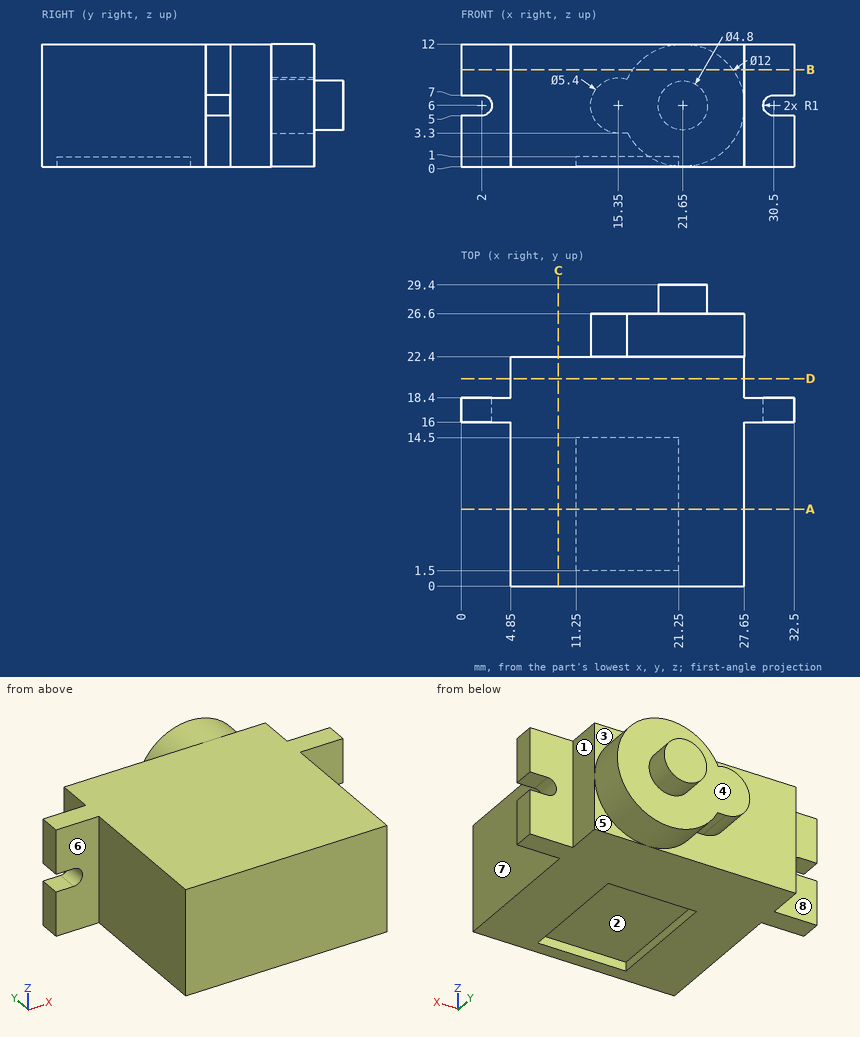
Study the drawing (mm; zero at the part's minimum x, y, z) and answer. A direction names the side the tool comes from. Coordinates: 2 decimals unless noted, no trailing zeros. Loops run counter-clockwise (first coordinate to the right, second up) from the corner with the lowest first, then second, coordinate; pieces in that order, holes last. Notation, with made-up numbers: M 69.5,74.5 L 124.5,74.5 A23 cw 124.5,106.5 Z; hole C 41.25,-24 d4. An arc over 180 degrees is marked long. Answer as a JSON object with one key per item and string values. Group by question number.
Item 1: Consider L1, parallel to Y at x = 16.5, z = 0.5; L2, parallel to Y at x = 14, z = 9.5; L3, parallel to Y at x = 17.5, z = 4. Determine where each line is inside the solid, lowest interval first.
Item 2: Each of these flat-tipped pins is pushed along its axis until it touches: P1, Ø1.8, axis at x = 25.5, z = 8.5, coming from the +Y side; P2, Ø5, axis at x = 22, z = 10, coming from the -Y side; P3, Ø5.5, axis at x = 3.5, z = 4.5, coming from the +Y side; P4, Ø1.5, axis at y = 21, z = 9, coming from the -X side. Where does it stop, or does it pass through?
Item 3: Section B-B (z = 9.5) is taken. Write down the section's boundary in (x, y), and give its area (3 significant figures).
Item 4: Section A-A (y = 7.5) is taken. Write down the section's boundary in (x, z), and give its area (3 significant figures).
Item 5: Section D-D (y = 20.25) is taken. Write down the section's boundary in (x, z).
Item 6: Determine the mould class of the marked faces 1, 2 and 3 for opening direction Y: +Y half, -Y half, draft (parallel to the pull), parting line (faces both ways), or undercut.
Item 7: Section C-C (x = 9.5) is taken. Write down the section's boundary in (y, z).
Item 8: Which of the six approach directions +Z, -Z, +X, -X, +Y, -Y give full straight-line access (tool end or side, diameter ignored) to the marked faces 4, 5, 6, 7 and 8?
Solved:
{
 "1": {"L1": "y = 0 to 1.5, 14.5 to 22.4", "L2": "y = 0 to 22.4", "L3": "y = 0 to 26.6"},
 "2": {"P1": "stops at y = 26.6", "P2": "stops at y = 0", "P3": "stops at y = 22.4", "P4": "stops at x = 4.85"},
 "3": {"outline": "M 0,16 L 4.85,16 L 4.85,0 L 27.65,0 L 27.65,16 L 32.5,16 L 32.5,18.4 L 27.65,18.4 L 27.65,22.4 L 26.52,22.4 L 26.52,26.6 L 16.78,26.6 L 16.78,22.4 L 4.85,22.4 L 4.85,18.4 L 0,18.4 Z", "area": "575 mm2"},
 "4": {"outline": "M 4.85,0 L 11.25,0 L 11.25,1 L 21.25,1 L 21.25,0 L 27.65,0 L 27.65,12 L 4.85,12 Z", "area": "264 mm2"},
 "5": {"outline": "M 4.85,0 L 27.65,0 L 27.65,12 L 4.85,12 Z"},
 "6": {"face 1": "draft", "face 2": "undercut", "face 3": "+Y half"},
 "7": {"outline": "M 0,0 L 22.4,0 L 22.4,12 L 0,12 Z"},
 "8": {"face 4": "+Y", "face 5": "-Z, +X, +Y", "face 6": "+Z, -Z, -X, -Y", "face 7": "+Z, -Z, +X, -Y", "face 8": "+Z, -Z, -X, +Y"}
}
